```python
from build123d import *

# Parameters (mm, degrees)
SKETCH1_R                = 19.05
SKETCH1_R_2              = 12.7
BOSS_EXTRUDE1_DEPTH      = 381
SKETCH2_R                = 50.8
SKETCH2_R_2              = 12.7
BOSS_EXTRUDE2_DEPTH      = 12.7
CUT_EXTRUDE1_DEPTH       = 388.714173071
CUT_EXTRUDE1_DEPTH_BACK  = 388.714173071
BOSS_EXTRUDE3_REACH      = 355.664
BOSS_EXTRUDE3_END_RADIUS = 19.05
BOSS_EXTRUDE3_START      = 31.75
SKETCH4_W                = 12.7
SKETCH4_H                = 12.7
SKETCH4_R                = 2.286


with BuildPart() as part:
    # Sketch1 → Boss-Extrude1 (new body)
    with BuildSketch(Plane(origin=(0, 0, 0), x_dir=(0, 0, -1), z_dir=(1, 0, 0))):
        Circle(SKETCH1_R)
        Circle(SKETCH1_R_2, mode=Mode.SUBTRACT)
    extrude(amount=-BOSS_EXTRUDE1_DEPTH)

    # Sketch2 → Boss-Extrude2 (add)
    with BuildSketch(Plane(origin=(0, 0, 0), x_dir=(0, 0, -1), z_dir=(1, 0, 0))):
        Circle(SKETCH2_R)
        Circle(SKETCH2_R_2, mode=Mode.SUBTRACT)
    extrude(amount=-BOSS_EXTRUDE2_DEPTH)

    # Sketch3 → Cut-Extrude1 (cut, two sides: drawn at the far end of the back side and taken through both)
    with BuildSketch(Plane(origin=(0, 0, 0), x_dir=(1, 0, 0), z_dir=(0, 1, 0)).offset(-CUT_EXTRUDE1_DEPTH_BACK)):
        Polygon((-330.049521684, 38.465573285), (-297.845785911, 0), (-308.119579729, -8.601315755), (-299.508024312, -18.88734028), (-330.049521684, -60.531095944), (-403.402475389, -60.531095944), (-403.402475389, 38.465573285), align=None)
    extrude(amount=CUT_EXTRUDE1_DEPTH + CUT_EXTRUDE1_DEPTH_BACK, mode=Mode.SUBTRACT)

    # Boss-Extrude3: up to this cylinder (the profile starts outside it)
    boss_extrude3_end = Plane(origin=(-25.4, 0, 0), z_dir=(1, 0, 0)) * Cylinder(BOSS_EXTRUDE3_END_RADIUS, 750.428, mode=Mode.PRIVATE)
    # Sketch4 → Boss-Extrude3 (add, up to the surface)
    with BuildSketch(Plane(origin=(0, 0, 0), x_dir=(1, 0, 0), z_dir=(0, 1, 0)).offset(BOSS_EXTRUDE3_START), mode=Mode.PRIVATE) as boss_extrude3_sk1:
        with Locations((-25.4, 0)):
            Rectangle(SKETCH4_W, SKETCH4_H)
        with Locations(Location((-25.4, 0, 0), (0, 0, 270))):
            Circle(SKETCH4_R, mode=Mode.SUBTRACT)
    boss_extrude3_tool1 = extrude(boss_extrude3_sk1.sketch, amount=-BOSS_EXTRUDE3_REACH, mode=Mode.PRIVATE) - boss_extrude3_end
    add(boss_extrude3_tool1.solids().sort_by_distance((-25.4, 31.75, 6.170395))[0])


solid = part.part
```
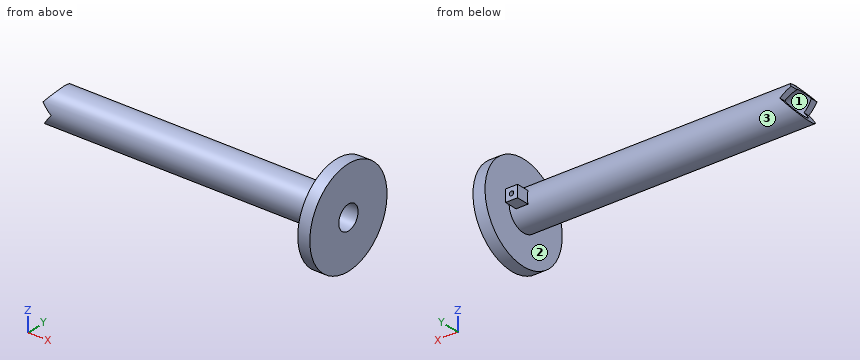
Source: CAD feature listing. Evaluate the final solid. Frame: model axes, mm. Face numbers are marked on the shaded views. Round coordinates to 2 decimals unless told otherwise and drop trailing zeros. Loops run counter-clockwise (first coordinate to the right, second up) from the corner with the lowest first, then second, coordinate; pieces in that order, holes last.
(1) Section query A-A (x = -189). Output: boundary loops of the cut face in (y, z), and give its area (3 significant figures).
From the geometry:
outline: circle Ø38.1 at (0, 0); hole circle Ø25.4 at (0, 0)
area: 633 mm2
(2) Section query D-D (y = -35). Output: boundary loops of the cut face in (x, z), and give its area (3 significant figures).
From the geometry:
outline: (-12.7, -36.82) - (0, -36.82) - (0, 36.82) - (-12.7, 36.82) - close
area: 935 mm2
(3) Pull-direction query (Z, two-part tool) for the marked faces 1, 2 and 3; classes: +Z half, -Z half, draft (parallel to the pull), parting line (faces both ways), or undercut.
From the geometry:
face 1: undercut
face 2: draft
face 3: parting line
(4) Contact query for flat-ended pins moving along their axis: pin 1 Ø3.5 at (x, z) = (-25.4, 0) entering from -Y; pin 2 Ø1 at (x, y) = (-160, -8.5) entering from +Z; pin 3 Ø5 at (x, z) = (-151.5, 7.5) entering from -Y. Output: stop coordinate, or through.
From the geometry:
pin 1: stops at y = -19.05
pin 2: stops at z = 17.29
pin 3: stops at y = -18.38
(5) Section query B-B (y = 5.5). Output: boundary loops of the cut face in (x, z), and give its area (3 significant figures).
From the geometry:
outline: (-313.12, -18.24) - (-12.7, -18.24) - (-12.7, -50.5) - (0, -50.5) - (0, -11.45) - (-307.43, -11.45) - close; (-305.74, 11.45) - (0, 11.45) - (0, 50.5) - (-12.7, 50.5) - (-12.7, 18.24) - (-300.05, 18.24) - close
area: 4,980 mm2
(6) Section query C-C (z = -34). Output: boundary loops of the cut face in (x, y).
From the geometry:
outline: (-12.7, -37.74) - (0, -37.74) - (0, 37.74) - (-12.7, 37.74) - close
(7) Material intervals for probe 1 along Z at (x, y) = (-25.4, 25); probe 2 along Z at (x, y) = (-105, 0), sorted ascending.
From the geometry:
probe 1: z = -6.35 to -2.29, 2.29 to 6.35
probe 2: z = -19.05 to -12.7, 12.7 to 19.05
